Check sheet for the drawn part. Datum: minimum x, y, z corner. Units: mm. A direction names the side the tool comes from. Give positions to 0.01 mm unless a question says otherwise; leave off trailing zeros.
(1) Thickness scan on line 1 along X through (y, z) = (3.5, 3.25) (1 decimal); line 2 along X through (y, z) = (3.25, 5.75); line 3 along X through (y, z) = (3.5, 4.25) (1 decimal). Record the ranges inside material, lowest first.
(2) Tool access check on the marked faces 3 and 4. Record the directions out of +Z, -Z, +X, -X, +Y, -Y that give a thin tool (end or side, any length) a straight path to the whole face; none if there is none.
(3) Cross-section at A-A (y = 4.75). Count the separate pieces of the cut face and the enclosed holes in it.
(4) Mould release check, pull along X, two halves, no side actions. Record for the marked faces 1 and 2: +X half, -X half, draft (parallel to the pull), parting line (faces both ways), or undercut.
(5) Depth check by flat-ended pin: P1, Ø3.5, axis at y = 5, z = 2.5, coming from the -X side; P2, Ø2.5, axis at y = 5, z = 4, coming from the +X side; P3, Ø2, axis at x = 24, z = 1, coming from the +Y side (3 decimals); P4, Ø3.5, axis at x = 63.373, z = 3.175, coming from the -Y side. Enter the tip coordinate at first touch or a pass-through.
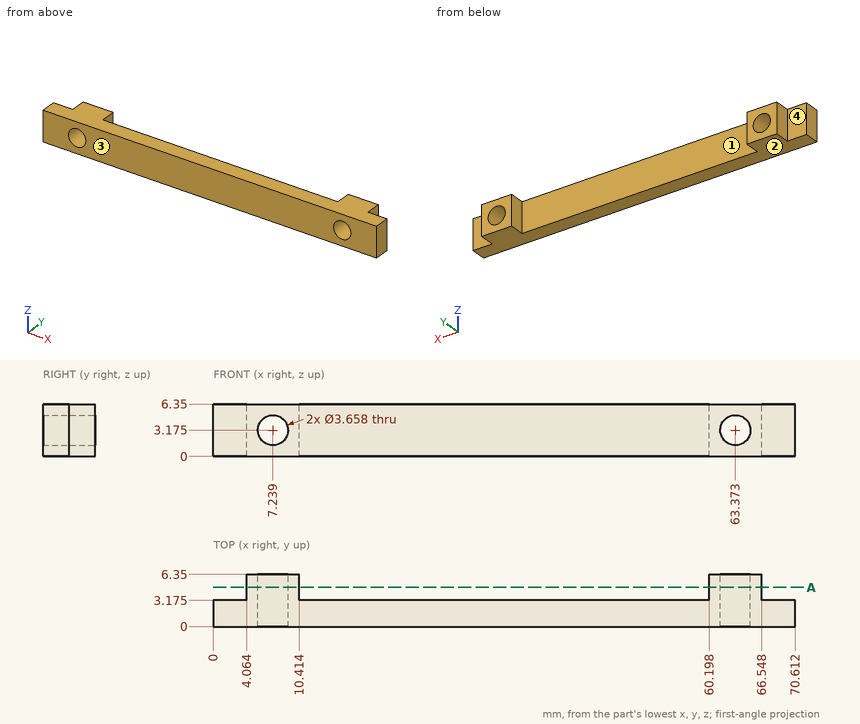
Reply:
1. line 1: x = 4.1 to 5.4, 9.1 to 10.4, 60.2 to 61.5, 65.2 to 66.5
1. line 2: x = 4.06 to 10.41, 60.2 to 66.55
1. line 3: x = 4.1 to 5.8, 8.7 to 10.4, 60.2 to 61.9, 64.9 to 66.5
2. face 3: +Z, -Z, +X, -X, -Y
2. face 4: +Z, -Z, -X, +Y
3. separate pieces: 2
3. enclosed holes: 2
4. face 1: undercut
4. face 2: draft
5. P1: stops at x = 4.06
5. P2: stops at x = 66.55
5. P3: stops at y = 3.175
5. P4: passes through
